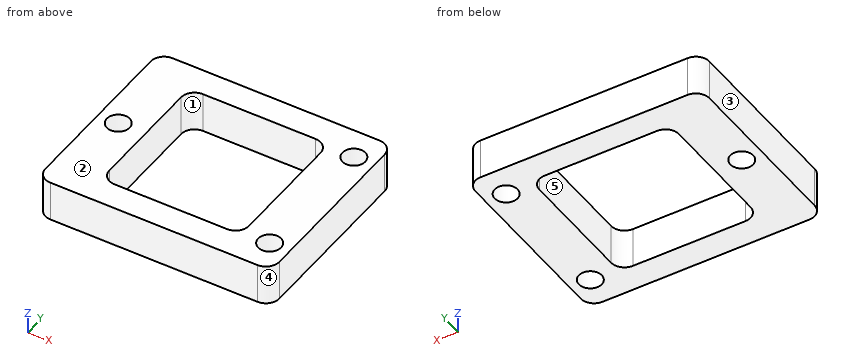
```python
from build123d import *

# Parameters (mm, degrees)
SKETCH_1_W          = 34.7
SKETCH_1_H          = 29
EXTRUDE_1_DEPTH     = 6
SKETCH_2_R          = 1.7
CUT_EXTRUDE_1_DEPTH = 25
SKETCH_3_W          = 20.7
SKETCH_3_H          = 21
CUT_EXTRUDE_2_DEPTH = 10
FILLET_1_R          = 2
FILLET_2_R          = 2


with BuildPart() as part:
    # 草图1 → 凸台-拉伸1 (new body)
    with BuildSketch(Plane.XY):
        Rectangle(SKETCH_1_W, SKETCH_1_H)
    extrude(amount=EXTRUDE_1_DEPTH)

    # 草图2 → 切除-拉伸1 (cut)
    with BuildSketch(Plane.XY.offset(6)):
        with Locations((14.35, -10)):
            Circle(SKETCH_2_R)
        with Locations((-14.35, 0)):
            Circle(SKETCH_2_R)
        with Locations((14.35, 10)):
            Circle(SKETCH_2_R)
    extrude(amount=-CUT_EXTRUDE_1_DEPTH, mode=Mode.SUBTRACT)

    # 草图3 → 切除-拉伸2 (cut)
    with BuildSketch(Plane.XY.offset(6)):
        Rectangle(SKETCH_3_W, SKETCH_3_H)
    extrude(amount=-CUT_EXTRUDE_2_DEPTH, mode=Mode.SUBTRACT)

    # 圆角1
    fillet_1_edges = [part.edges().sort_by_distance(p)[0] for p in [
        (10.35, 10.5, 3),
        (10.35, -10.5, 3),
        (-10.35, -10.5, 3),
        (-10.35, 10.5, 3),
    ]]
    fillet(fillet_1_edges, radius=FILLET_1_R)

    # 圆角2
    fillet_2_edges = [part.edges().sort_by_distance(p)[0] for p in [
        (17.35, -14.5, 3),
        (-17.35, -14.5, 3),
        (-17.35, 14.5, 3),
        (17.35, 14.5, 3),
    ]]
    fillet(fillet_2_edges, radius=FILLET_2_R)


solid = part.part
```
Could you check a few things on this model? Use its own coordinates, in mm. Face numbers are marked on the shaded views. A direction names the side the tool comes from. Coordinates: 2 decimals unless noted, no trailing zeros. Write each loop counter-clockwise with the first axis right and the second up, starting at its lowest first coordinate (ties: lowest second). Pieces come first, ordered by that corner, then holes. Notation, with made-up numbers: M 37,-7.75 L 60,-7.75 A17 cw 60,-1.75 Z; hole C 14,54 d8. An arc over 180 degrees is marked long. Answer as CSV lines item,"result". Start each with the question number.
1) For P1, Ø2, axis at x = -14.35, y = 0, coming from the +Z side (3 decimals); P2, Ø4, axis at x = 14.35, y = 10, coming from the -Z side, each with a flat end and sliding along its axis, tell me the tip position at first contact or that it passes through.
2) I want a section at C-C, the plane x = 14.35. Please give me the cut outline in (y, z), and give its area (3 significant figures).
3) For the marked faces 4 and 5, which set-ups out of +Z, -Z, +X, -X, +Y, -Y let a thin tool reach every point of the face, with its end or its side?
4) We'd pull the mould along X, two halves only. Please class the marked faces 1, 2 and 3: +X half, -X half, draft (parallel to the pull), parting line (faces both ways), or undercut.
5) I want a section at D-D, the plane z = 4.9. Please give me the cut outline in (x, y).
6) I want a section at A-A, the plane y = 0. Please give me the cut outline in (x, z).
7) Please list where these lines run through material, in increasing order: line 1 (Y direction, x = 14.35, z = 4.4); line 2 (Y direction, x = -3, z = 4.8); line 3 (X direction, y = -7, z = 0.85). Write a range as from..to.
8) I want a section at B-B, the plane x = 5.5. Please give me the cut outline in (y, z), and give its area (3 significant figures).
Data:
1,P1,"passes through"
1,P2,"stops at z = 0"
2,outline,"M -14.5,0 L -11.7,0 L -11.7,6 L -14.5,6 Z; M -8.3,0 L 8.3,0 L 8.3,6 L -8.3,6 Z; M 11.7,0 L 14.5,0 L 14.5,6 L 11.7,6 Z"
2,area,"133 mm^2"
3,face 4,"+Z, -Z, +X, -Y"
3,face 5,"+Z, -Z"
4,face 1,"undercut"
4,face 2,"draft"
4,face 3,"-X half"
5,outline,"M -17.35,-12.5 A2 ccw -15.35,-14.5 L 15.35,-14.5 A2 ccw 17.35,-12.5 L 17.35,12.5 A2 ccw 15.35,14.5 L -15.35,14.5 A2 ccw -17.35,12.5 Z; hole C -14.35,0 d3.4; hole M -10.35,-8.5 A2 ccw -8.35,-10.5 L 8.35,-10.5 A2 ccw 10.35,-8.5 L 10.35,8.5 A2 ccw 8.35,10.5 L -8.35,10.5 A2 ccw -10.35,8.5 Z; hole C 14.35,-10 d3.4; hole C 14.35,10 d3.4"
6,outline,"M -17.35,0 L -16.05,0 L -16.05,6 L -17.35,6 Z; M -12.65,0 L -10.35,0 L -10.35,6 L -12.65,6 Z; M 10.35,0 L 17.35,0 L 17.35,6 L 10.35,6 Z"
7,line 1,"y = -14.5..-11.7, -8.3..8.3, 11.7..14.5"
7,line 2,"y = -14.5..-10.5, 10.5..14.5"
7,line 3,"x = -17.35..-10.35, 10.35..17.35"
8,outline,"M -14.5,0 L -10.5,0 L -10.5,6 L -14.5,6 Z; M 10.5,0 L 14.5,0 L 14.5,6 L 10.5,6 Z"
8,area,"48.0 mm^2"
